Check sheet for the drawn part. Datum: minimum x, y, z corner. Units: mm. A direction names the side the tool comes from. Coordinates: 2 decimals unless noted, no trailing zeros. Write each loop counter-clockwise with the first axis right and the second up, starting at its lowest first coordinate (ties: lowest second). Pieces come first, ordered by that corner, then holes. Notation, with made-up numbers: M 50.25,75.25 L 78.25,75.25 A21 ccw 78.25,88.25 Z; hole C 88.25,80.5 d2. An arc over 180 degrees is marked long. Answer in a Markdown table with one row per item.
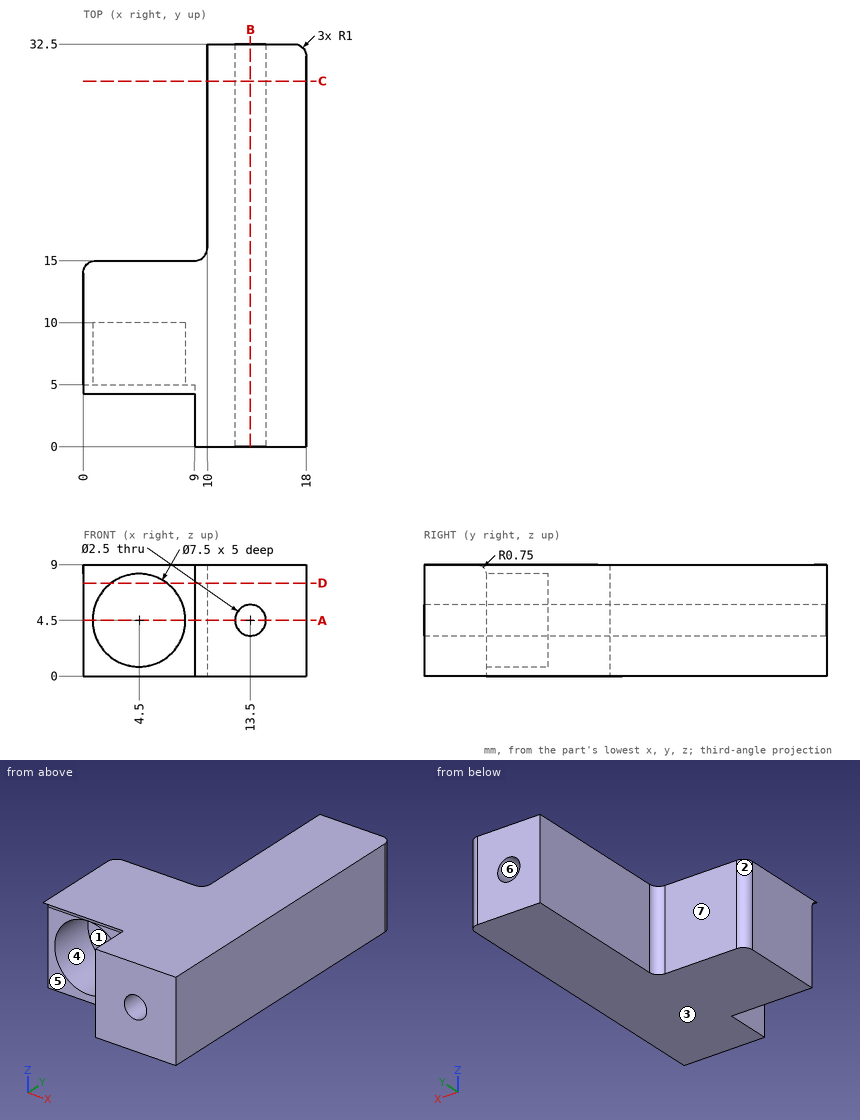
1) Sectioned sample at D-D (z = 7.5). Record the cut outline in (x, y), then the cut area to 3 significant figures.
Response values:
| item | result |
|---|---|
| outline | M 0,5 L 2.25,5 L 2.25,10 L 6.75,10 L 6.75,5 L 9,5 L 9,0 L 18,0 L 18,31.5 A1 ccw 17,32.5 L 10,32.5 L 10,16 A1 cw 9,15 L 1,15 A1 ccw 0,14 Z |
| area | 342 mm² |
2) Release check for a two-part mould opening along Z. For the marked faces 1, 2 and 3 record: +Z half, -Z half, draft (parallel to the pull), parting line (faces both ways), or undercut.
Response values:
| item | result |
|---|---|
| face 1 | undercut |
| face 2 | draft |
| face 3 | -Z half |
3) Sectioned sample at A-A (z = 4.5). Record the cut outline in (x, y), then the cut area to 3 significant figures.
Response values:
| item | result |
|---|---|
| outline | M 0,5 L 0.75,5 L 0.75,10 L 8.25,10 L 8.25,5 L 9,5 L 9,0 L 12.25,0 L 12.25,32.5 L 10,32.5 L 10,16 A1 cw 9,15 L 1,15 A1 ccw 0,14 Z; M 14.75,0 L 18,0 L 18,31.5 A1 ccw 17,32.5 L 14.75,32.5 Z |
| area | 246 mm² |
4) Depth check by flat-ended pin: pin 1 (3 mm diameter, centred on y = 21.5, z = 1, fed in from -X); pin 2 (1 mm diameter, centred on x = 5, z = 8, fed in from -Y); pin 3 (4 mm diameter, centred on x = 5, z = 5, fed in from -Y); pin 4 (4 mm diameter, centred on x = 13.5, z = 4.5, fed in from +Y). Enter the tip coordinate at first touch or a pass-through.
Response values:
| item | result |
|---|---|
| pin 1 | stops at x = 10 |
| pin 2 | stops at y = 4.96 |
| pin 3 | stops at y = 10 |
| pin 4 | stops at y = 32.5 |
5) Tool access check on the marked faces 4, 5, 6 and 7. Record the directions out of +Z, -Z, +X, -X, +Y, -Y that give a thin tool (end or side, any length) a straight path to the whole face; none if there is none.
Response values:
| item | result |
|---|---|
| face 4 | -Y |
| face 5 | -Z, -X, -Y |
| face 6 | +Y, -Y |
| face 7 | +Z, -Z, -X, +Y |
6) Sectioned sample at B-B (x = 13.5). Record the cut outline in (y, z), then the cut area to 3 significant figures.
Response values:
| item | result |
|---|---|
| outline | M 0,0 L 32.5,0 L 32.5,3.25 L 0,3.25 Z; M 0,5.75 L 32.5,5.75 L 32.5,9 L 0,9 Z |
| area | 211 mm² |
7) Thickness scan on L1, parallel to X at y = 7.7, z = 4.5; L2, parallel to X at y = 13, z = 4.5; L3, parallel to X at y = 20.5, z = 4.5. Record the ranges inside material, lowest first. Write a range as [from, to].
Response values:
| item | result |
|---|---|
| L1 | x = [0, 0.75], [8.25, 12.25], [14.75, 18] |
| L2 | x = [0, 12.25], [14.75, 18] |
| L3 | x = [10, 12.25], [14.75, 18] |
8) Sectioned sample at C-C (y = 29.5). Record the cut outline in (x, z).
Response values:
| item | result |
|---|---|
| outline | M 10,0 L 18,0 L 18,9 L 10,9 Z; hole C 13.5,4.5 d2.5 |
